```python
from build123d import *

# Parameters (mm, degrees)
F0_W     = 400
F0_H     = 200
F1_DEPTH = 20
F2_R     = 75
F2_R_2   = 60
F3_DEPTH = 25
F4_W     = 5
F4_H     = 10
F5_DEPTH = 10


with BuildPart() as f1:
    # F0 (on Top) → F1 (new body)
    with BuildSketch(Plane.XY):
        Rectangle(F0_W, F0_H)
    extrude(amount=F1_DEPTH)

    # F2 (on face) → F3 (join)
    with BuildSketch(Plane.XY.offset(20)):
        with Locations((-120, 0)):
            Circle(F2_R)
        with Locations((-120, 0)):
            Circle(F2_R_2, mode=Mode.SUBTRACT)
    extrude(amount=F3_DEPTH)

    # F4 (on face) → F5 (cut)
    with BuildSketch(Plane.XY.offset(20)):
        with Locations((-182.5, -70)):
            Rectangle(F4_W, F4_H)
    extrude(amount=-F5_DEPTH, mode=Mode.SUBTRACT)


solid = f1.part
```
Input: part model. Units: mm. Frame: model coordinates. A direction names the side the tool comes from. Coordinates: 2 decimals unless noted, no trailing zeros. Loops run counter-clockwise (first coordinate to the right, second up) from the corner with the lowest first, then second, coordinate; pieces in that order, holes last. Notation, with made-up numbers: M -14,-16.5 L 16,-16.5 A4 cw 16,-11.5 Z; hole C 22.25,-20 d7. An arc over 180 degrees is marked long. One line per item, written item: value.
(1) Section A-A (y = 0). Output: boundary loops of the cut face in (x, z), and give its area (3 significant figures).
Filled in:
outline: M -200,0 L 200,0 L 200,20 L -45,20 L -45,45 L -60,45 L -60,20 L -180,20 L -180,45 L -195,45 L -195,20 L -200,20 Z
area: 8,750 mm^2
(2) Pin query (flat end, axial travel): pin 1 (1 mm diameter, centred on y = -6, z = 29.5, fed in from +X); pin 2 (5.5 mm diameter, centred on x = -183, y = -69, fed in from +Z). Return the tip coordinate at first contact, or that it passes through.
Filled in:
pin 1: x = -45.2
pin 2: z = 20
(3) Section B-B (x = -110.5). Output: boundary loops of the cut face in (y, z), and give its area (3 significant figures).
Filled in:
outline: M -100,0 L 100,0 L 100,20 L 74.4,20 L 74.4,45 L 59.24,45 L 59.24,20 L -59.24,20 L -59.24,45 L -74.4,45 L -74.4,20 L -100,20 Z
area: 4,760 mm^2
(4) Pull-direction query (X, two-part tool) for faces 3 (the flat face through (42, 1, 20)), 4 (the flat face through (-200, -1, 10)), 5 (the cylindrical face through (-179.94, 2.64, 32.33)); classes: +X half, -X half, draft (parallel to the pull), parting line (faces both ways), or undercut.
Filled in:
face 3: draft
face 4: -X half
face 5: undercut
(5) Section D-D (x = -36). Output: boundary loops of the cut face in (y, z), and give its area (3 significant figures).
Filled in:
outline: M -100,0 L 100,0 L 100,20 L -100,20 Z
area: 4,000 mm^2
(6) Reachability of faces 1 (the flat face through (200, -1, 10)), 2 (the flat face through (-121, 1, 20)) from +Z, -Z, +X, -X, +Y, -Y: full face, straight path, thin tool, end or side. Return the list, or none.
Filled in:
face 1: +Z, -Z, +X, +Y, -Y
face 2: +Z
(7) Section C-C (z = 35). Output: boundary loops of the cut face in (x, y).
Filled in:
outline: C -120,0 d150; hole C -120,0 d120
(8) Line query: line 1 along Y through (x, z) = (-120, 34); line 2 along Z through (x, y) = (134.5, -41.5); line 3 along Y through (x, z) = (-101, 25). Output: solid intervals per line, ascending. Write a range as from..to.
Filled in:
line 1: -75..-60, 60..75
line 2: 0..20
line 3: -72.55..-56.91, 56.91..72.55
